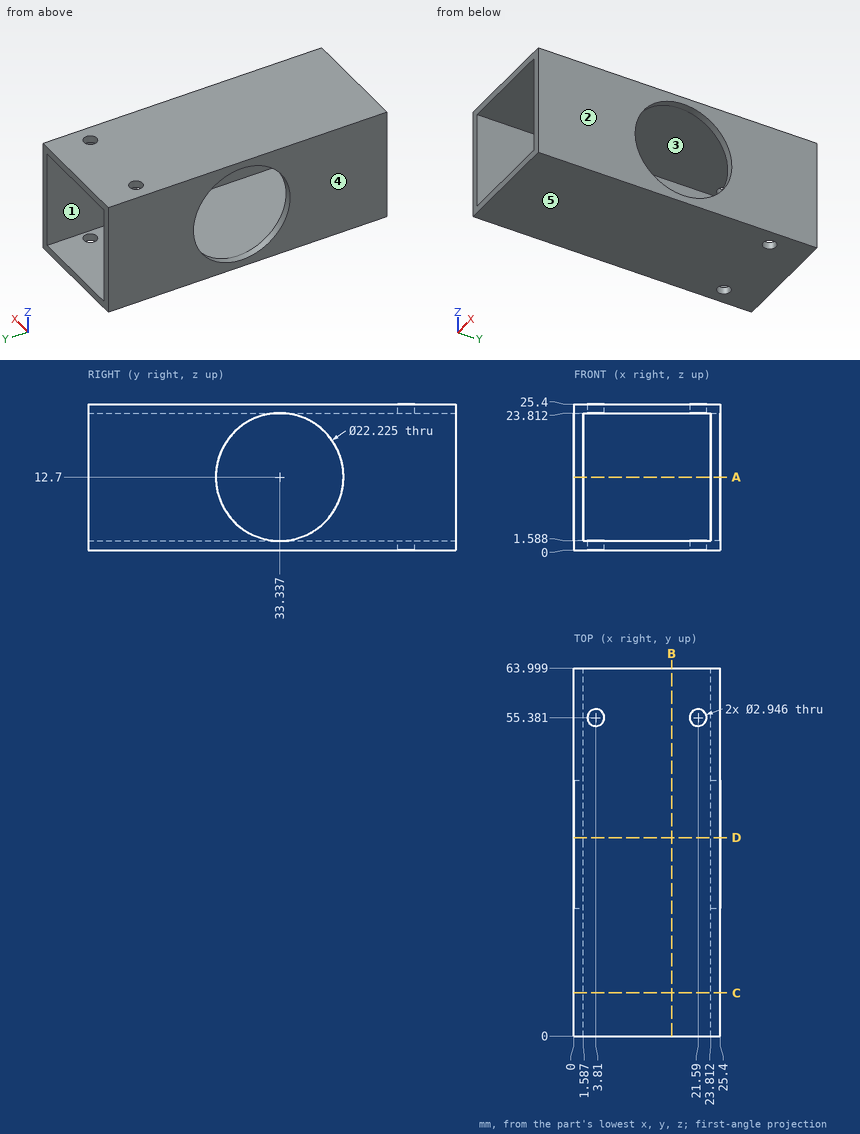
Geometry: see drawing. Coordinates: mm, zero at the bounding-box minimum. A direction names the side the tool comes from. Coordinates: 2 decimals unless noted, no trailing zeros. Write each loop counter-clockwise with the first axis right and the second up, starting at its lowest first coordinate (ties: lowest second). Pieces come first, ordered by that corner, then holes. Notation, with made-up numbers: M 37.5,84 L 64.5,84 A19 ccw 64.5,111 Z; hole C -1.75,15 d3. An arc over 180 degrees is marked long. Answer as a JSON object with one key per item and string values.
1. Cut plane B-B on x = 17. Output: boundary loops of the cut face in (y, z).
Evaluation:
{"outline": "M 0,0 L 64,0 L 64,1.59 L 0,1.59 Z; M 0,23.81 L 64,23.81 L 64,25.4 L 0,25.4 Z"}
2. Cut plane A-A on z = 12.7. State how many separate pieces and enclosed holes the cut face has.
Evaluation:
{"separate pieces": "4", "enclosed holes": "0"}
3. Contact query for a flat-ended pin moving along its axis: P1, Ø4, axis at x = 3.81, y = 55.38, coming from the +Z side. Output: stop coordinate, or through.
Evaluation:
{"P1": "z = 25.4"}
4. Ray query, L1, parallel to X at y = 55, z = 12.5; L2, parallel to Y at x = 1, z = 4.5 (1 decimal). Return the intervals inside material, ascending.
Evaluation:
{"L1": "0 to 1.59, 23.81 to 25.4", "L2": "0 to 25.8, 40.8 to 64"}
5. Draft query along Z for the marked faces 3, 4 and 5. Return one class per face: released by +Z, released by -Z, zero draft, split by the parting line, or undercut.
Evaluation:
{"face 3": "undercut", "face 4": "zero draft", "face 5": "released by -Z"}
6. Access query for the marked faces 1 and 2. Directions: +Z, -Z, +X, -X, +Y, -Y. A direction counts if a zero-diameter tool reaches every point of the face in a straight line with its end or side. Return the directions, or none.
Evaluation:
{"face 1": "+Y, -Y", "face 2": "+Z, -Z, +X, +Y, -Y"}
7. Cut plane D-D on y = 34.5. Output: boundary loops of the cut face in (x, z).
Evaluation:
{"outline": "M 0,0 L 25.4,0 L 25.4,1.65 L 23.81,1.65 L 23.81,1.59 L 1.59,1.59 L 1.59,1.65 L 0,1.65 Z; M 0,23.75 L 1.59,23.75 L 1.59,23.81 L 23.81,23.81 L 23.81,23.75 L 25.4,23.75 L 25.4,25.4 L 0,25.4 Z"}
8. Cut plane C-C on y = 7.5. Output: boundary loops of the cut face in (x, z), plus the area to 3 significant figures.
Evaluation:
{"outline": "M 0,0 L 25.4,0 L 25.4,25.4 L 0,25.4 Z; hole M 1.59,1.59 L 23.81,1.59 L 23.81,23.81 L 1.59,23.81 Z", "area": "151 mm^2"}
